Autodesk Inventor part; units mm, degrees
ref_plane "C1_XY" through (0, 0, 0) normal (1, 0, 0) x (0, 0, -1)
ref_plane "C1_YZ" through (0, 0, 0) normal (0, 0, -1) x (0, 1, 0)
ref_plane "C1_ZX" through (0, 0, 0) normal (0, 1, 0) x (1, 0, 0)
sketch "Skizze_1" plane through (0, 0, 0) normal (0, 0, 1) x (1, 0, 0)
  line L0 (77, 0) -> (-17, 0)
  line L1 (-17, 0) -> (-17, 7.08)
  line L2 (-17, 7.08) -> (-15, 7.08)
  line L3 (-15, 7.08) -> (-14.08, 8)
  line L4 (-14.08, 8) -> (0, 8)
  line L5 (0, 8) -> (0, 10)
  line L6 (0, 10) -> (9, 10)
  line L7 (9, 10) -> (9, 6.5)
  line L8 (9, 6.5) -> (9.5, 7)
  line L9 (9.5, 7) -> (50.5, 7)
  line L10 (50.5, 7) -> (51, 6.5)
  line L11 (51, 6.5) -> (51, 10)
  line L12 (51, 10) -> (60, 10)
  line L13 (60, 10) -> (60, 8)
  line L14 (60, 8) -> (76.08, 8)
  line L15 (76.08, 8) -> (77, 7.08)
  line L16 (77, 7.08) -> (77, 0)
  line L17 (77, 0) -> (-17, 0)
revolve "Revolution1" add sketch "Skizze_1" angle 360 about axis through (77, 0, 0) along (1, 0, 0)
thread "Thread1"
thread "Thread2"
sketch "Skizze_3" plane through (0, 0, 0) normal (1, 0, 0) x (0, 1, 0)
  line L0 (10.5, 5.5) -> (0, 5.5)
  line L1 (0, 5.5) -> (0, -5.5)
  line L2 (0, -5.5) -> (10.5, -5.5)
  line L3 (10.5, -5.5) -> (10.5, 5.5)
extrude "Extrusion1" add sketch "Skizze_3" along normal blind 9
sketch "Skizze_4" plane through (60, 0, 0) normal (1, 0, 0) x (0, 0, -1)
  line L0 (-5.5, 10.5) -> (-5.5, 0)
  line L1 (-5.5, 0) -> (5.5, 0)
  line L2 (5.5, 0) -> (5.5, 10.5)
  line L3 (5.5, 10.5) -> (-5.5, 10.5)
extrude "Extrusion2" add sketch "Skizze_4" against normal blind 9
sketch "Skizze_16_ALT_Drilling_1" plane through (0, 0, 0) normal (0, 0, 1) x (1, 0, 0)
  line L0 (51, 0) -> (-17, 0)
  line L1 (-17, 0) -> (-17, 3)
  line L2 (-17, 3) -> (38, 3)
  line L3 (38, 3) -> (38, 5.6)
  line L4 (38, 5.6) -> (51, 5.6)
  line L5 (51, 5.6) -> (51, 0)
  line L6 (51, 0) -> (-17, 0)
revolve "Revolution2" cut sketch "Skizze_16_ALT_Drilling_1" angle 360 about axis through (51, 0, 0) along (1, 0, 0)
sketch "Skizze_7" plane through (0, 0, 0) normal (0, 1, 0) x (-1, 0, 0)
  line L0 (-54, -12) -> (-54, -6)
  line L1 (-54, -6) -> (-77, -6)
  line L2 (-77, -6) -> (-77, 6)
  line L3 (-77, 6) -> (-54, 6)
  line L4 (-54, 6) -> (-54, 12)
  line L5 (-54, 12) -> (-86, 12)
  line L6 (-86, 12) -> (-86, -12)
  line L7 (-86, -12) -> (-54, -12)
extrude "Extrusion3" cut sketch "Skizze_7" along normal mid plane 24
sketch "Skizze_8" plane through (0, 0, 0) normal (0, 0, 1) x (1, 0, 0)
  circle A0 centre (63, 0) radius 3
extrude "Extrusion4" cut sketch "Skizze_8" along normal mid plane 24
sketch "Skizze_9_ALT_Drilling_2" plane through (0, 0, 0) normal (0, 0, 1) x (1, 0, 0)
  line L0 (4.5, 10.5) -> (4.5, 5.3398)
  line L1 (4.5, 5.3398) -> (2.4905, 6.5)
  line L2 (2.4905, 6.5) -> (2.4905, 10.0095)
  line L3 (2.4905, 10.0095) -> (2, 10.5)
  line L4 (2, 10.5) -> (4.5, 10.5)
  line L5 (4.5, 10.5) -> (4.5, 5.3398)
revolve "Revolution3" cut sketch "Skizze_9_ALT_Drilling_2" angle 360 about axis through (4.5, 10.5, 0) along (0, 1, 0)
sketch "Skizze_10_ALT_Drilling_3" plane through (0, 0, 0) normal (0, 0, 1) x (1, 0, 0)
  line L0 (55.5, 10.5) -> (55.5, 5.3398)
  line L1 (55.5, 5.3398) -> (53.4905, 6.5)
  line L2 (53.4905, 6.5) -> (53.4905, 10.0095)
  line L3 (53.4905, 10.0095) -> (53, 10.5)
  line L4 (53, 10.5) -> (55.5, 10.5)
  line L5 (55.5, 10.5) -> (55.5, 5.3398)
revolve "Revolution4" cut sketch "Skizze_10_ALT_Drilling_3" angle 360 about axis through (55.5, 10.5, 0) along (0, 1, 0)
ref_plane "C1_XY" through (0, 0, 0) normal (1, 0, 0) x (0, 0, -1)
ref_plane "C1_YZ" through (0, 0, 0) normal (0, 0, -1) x (0, 1, 0)
ref_plane "C1_ZX" through (0, 0, 0) normal (0, 1, 0) x (1, 0, 0)
ref_plane "CD1_XY" through (0, 0, 0) normal (1, 0, 0) x (0, 0, -1)
ref_plane "CD1_YZ" through (0, 0, 0) normal (0, 0, -1) x (0, 1, 0)
ref_plane "CD1_ZX" through (0, 0, 0) normal (0, 1, 0) x (1, 0, 0)
ref_plane "CD2_XY" through (60, 0, 0) normal (1, 0, 0) x (0, 0, -1)
ref_plane "CD2_YZ" through (60, 0, 0) normal (0, 0, -1) x (0, 1, 0)
ref_plane "CD2_ZX" through (60, 0, 0) normal (0, 1, 0) x (1, 0, 0)
ref_plane "RL_XY" through (-17, 0, 0) normal (1, 0, 0) x (0, 0, -1)
ref_plane "RL_YZ" through (-17, 0, 0) normal (0, 0, -1) x (0, 1, 0)
ref_plane "RL_ZX" through (-17, 0, 0) normal (0, 1, 0) x (1, 0, 0)
properties part number "16N2A12A010-(N0-cilindro)"
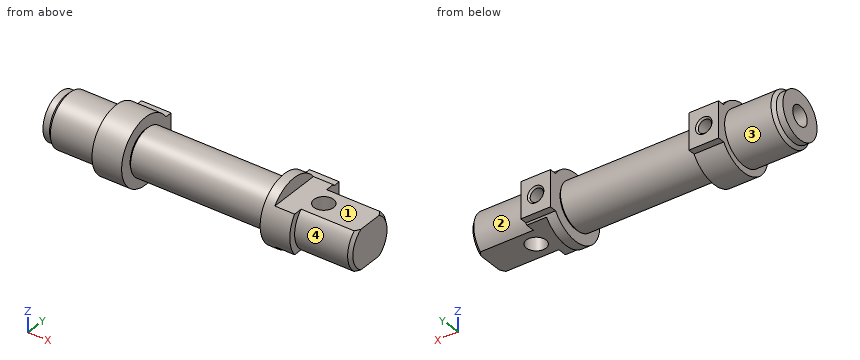
CAD build for the part. Positions are in the model's coordinates, mm. Face numbers are marked on the shaded views. A direction names the side the tool comes from. Round coordinates to 2 decimals unless told otherwise and drop trailing zeros. Order: outer loops, then holes, each group sorted by start corner. A loop starts at its lowest first (then second) coordinate and runs counter-clockwise, first axis right, second up. Notation, with made-up numbers: (53.25, -5.5) - (107.25, -5.5) arc R38 ccw to (107.25, 33.5) - close; hole circle Ø1 at (86, 47.5). An arc over 180 degrees is marked (long way). Use CSV: the item, a comma, the result in double quotes. Start each with the question number.
1) Saw through at B-B (x = 32.5). List the corners of the cut face in (y, z).
2) Saw through at D-D (z = 4). Count the separate pieces of the cut face and the enclosed holes in it, and give its area (3 significant figures).
3) Pin check, flat tips, straight feed: pin 1 Ø1.7 at (x, y) = (6, 9.5) entering from -Z; pin 2 Ø2 at (x, y) = (-2.5, -0.5) entering from -Z; pin 3 Ø8 at (x, y) = (65, -2) entering from -Z; pin 4 Ø3.5 at (x, y) = (63, 0) entering from +Z. Stop position of each tip, or through.
4) Tool access for the marked faces 1, 2, 3 and 4: list every direction of +Z, -Z, +X, -X, +Y, -Y with a clear straight run to the whole face (end or side of a thin tool).
5) Saw through at C-C (x = 47.5). List the corners of the cut face in (y, z), and give its area (3 significant figures).
6) Saw through at A-A (x = 63). List the corners of the cut face in (y, z).
7) Wall check: L1, parallel to X at y = 0, z = -3.25; L2, parallel to X at y = 0, z = -1.5; L3, parallel to X at y = -4.5, z = -8. Give the ranges that are in metal, low to high. Write a range as [from, to].
Values follow:
1,outline,"circle Ø14 at (0, 0); hole circle Ø6 at (0, 0)"
2,separate pieces,"1"
2,enclosed holes,"2"
2,area,"1,170 mm2"
3,pin 1,"stops at z = -5.5"
3,pin 2,"stops at z = -8"
3,pin 3,"stops at z = -6"
3,pin 4,"passes through"
4,face 1,"+Z, +X, +Y, -Y"
4,face 2,"+X, +Y"
4,face 3,"-X"
4,face 4,"+X, -Y"
5,outline,"circle Ø14 at (0, 0); hole circle Ø11.2 at (0, 0)"
5,area,"55.4 mm2"
6,outline,"(-5.29, -6) - (-3, -6) - (-3, 6) - (-5.29, 6) arc R8 ccw to start; (3, -6) - (5.29, -6) arc R8 ccw to (5.29, 6) - (3, 6) - close"
7,L1,"x = [-17, 38], [51, 60], [66, 77]"
7,L2,"x = [51, 60], [66, 77]"
7,L3,"x = [0, 9], [51, 54]"
